The listing builds one solid part. Answer for the finished solid, in the listing's coordinates (mm). Face numbers are marked on the shaded views. A direction names the side the tool comes from. Give positions to 0.01 mm unless a question says otherwise; leave off trailing zeros. Write each loop counter-clockwise with the first axis right and the second up, starting at its lowest first coordinate (ties: lowest second). Pieces come first, ordered by that corner, then holes. Notation, with made-up numbers: (-37.75, 48) -> (-22.75, 48) arc R29 cw to (-22.75, 81) -> close; hole circle Ø2 at (44.5, 2). An arc over 180 degrees is marked (long way). Use CSV: the item, a comma, the result in double quotes. Start each with the question number.
from build123d import *

# Parameters (mm, degrees)
BOSS_EXTRUDE1_DEPTH = 7.5
FILLET1_R           = 5
SKETCH2_W           = 7.7
SKETCH2_H           = 14.7
BOSS_EXTRUDE2_DEPTH = 100
SKETCH3_R           = 2.5
CUT_EXTRUDE1_DEPTH  = 100
SKETCH4_W           = 15
SKETCH4_H           = 60
CUT_EXTRUDE2_DEPTH  = 100
CUT_EXTRUDE3_DEPTH  = 3.75
BOSS_EXTRUDE3_DEPTH = 3.75
SKETCH10_W          = 2.5
SKETCH10_H          = 90
CUT_EXTRUDE4_DEPTH  = 199.475521198


with BuildPart() as part:
    # Sketch1 → Boss-Extrude1 (new, symmetric)
    with BuildSketch(Plane.XY):
        with BuildLine():
            Line((15, 99.936708861), (15, -115.063291139))
            ThreePointArc((15, -115.063291139), (0, -130.063291139), (-15, -115.063291139))
            Line((-15, -115.063291139), (-15, 124.936708861))
            ThreePointArc((-15, 124.936708861), (0, 139.936708861), (15, 124.936708861))
            Line((15, 124.936708861), (25, 124.936708861))
            Line((25, 124.936708861), (25, 99.936708861))
            Line((25, 99.936708861), (15, 99.936708861))
        make_face()
    extrude(amount=BOSS_EXTRUDE1_DEPTH, both=True)

    # Fillet1
    fillet1_edges = [part.edges().sort_by_distance(p)[0] for p in [
        (0, 139.936708861, -7.5),
        (0, -130.063291139, 7.5),
        (15, -7.563291139, 7.5),
        (20, 99.936708861, 7.5),
        (20, 124.936708861, 7.5),
        (0, 139.936708861, 7.5),
        (20, 124.936708861, -7.5),
        (20, 99.936708861, -7.5),
        (15, -7.563291139, -7.5),
        (-15, 4.936708861, 7.5),
        (0, -130.063291139, -7.5),
        (-15, 4.936708861, -7.5),
    ]]
    fillet(fillet1_edges, radius=FILLET1_R)

    # Sketch2 → Boss-Extrude2 (add)
    with BuildSketch(Plane(origin=(25, 0, 0), x_dir=(0, 0, -1), z_dir=(1, 0, 0))):
        with Locations((0, 112.436708861)):
            Rectangle(SKETCH2_W, SKETCH2_H)
    extrude(amount=BOSS_EXTRUDE2_DEPTH)

    # Sketch3 → Cut-Extrude1 (cut)
    with BuildSketch(Plane.XY.offset(3.85)):
        with Locations((35, 112.336708861)):
            Circle(SKETCH3_R)
        with Locations((55, 112.336708861)):
            Circle(SKETCH3_R)
        with Locations((75, 112.336708861)):
            Circle(SKETCH3_R)
        with Locations((95, 112.336708861)):
            Circle(SKETCH3_R)
        with Locations((115, 112.336708861)):
            Circle(SKETCH3_R)
    extrude(amount=-CUT_EXTRUDE1_DEPTH, mode=Mode.SUBTRACT)

    # Sketch4 → Cut-Extrude2 (cut)
    with BuildSketch(Plane.XY.offset(7.5)):
        with Locations((0, -100.063291139)):
            Rectangle(SKETCH4_W, SKETCH4_H)
    extrude(amount=-CUT_EXTRUDE2_DEPTH, mode=Mode.SUBTRACT)

    # Sketch7 → Cut-Extrude3 (cut, symmetric)
    with BuildSketch(Plane(origin=(0, 0, 0), x_dir=(0, 0, -1), z_dir=(1, 0, 0))):
        Polygon((0, 69.936708861), (-7.5, 64.685152324), (-7.5, 74.685152324), (0, 79.936708861), align=None)
        Polygon((0, 49.936708861), (0, 59.936708861), (-7.5, 54.685152324), (-7.5, 44.685152324), align=None)
        Polygon((0, 29.936708861), (0, 39.936708861), (-7.5, 34.685152324), (-7.5, 24.685152324), align=None)
    extrude(amount=CUT_EXTRUDE3_DEPTH, both=True, mode=Mode.SUBTRACT)

    # Sketch8 → Revolve1 (revolve)
    with BuildSketch(Plane.XY):
        with BuildLine():
            Line((-7.5, -113.063291139), (-6, -113.063291139))
            ThreePointArc((-6, -113.063291139), (-6.439339828, -112.002630967), (-7.5, -111.563291139))
            Line((-7.5, -111.563291139), (-7.5, -113.063291139))
        make_face()
        with BuildLine():
            Line((7.5, -113.063291139), (6, -113.063291139))
            ThreePointArc((6, -113.063291139), (6.439339828, -112.002630967), (7.5, -111.563291139))
            Line((7.5, -111.563291139), (7.5, -113.063291139))
        make_face()
    revolve(axis=Axis((-28.138828416, -113.063291139, 0), (1, 0, 0)))

    # Sketch9 → Boss-Extrude3 (add, symmetric)
    with BuildSketch(Plane(origin=(0, 0, 0), x_dir=(0, 0, -1), z_dir=(1, 0, 0))):
        with BuildLine():
            Line((-7.5, 89.436708861), (-7.5, 97.436708861))
            Line((-7.5, 97.436708861), (-14.5, 97.436708861))
            Line((-14.5, 97.436708861), (-14.5, 92.436708861))
            Line((-14.5, 92.436708861), (-10.5, 92.436708861))
            ThreePointArc((-10.5, 92.436708861), (-8.378679656, 91.558029204), (-7.5, 89.436708861))
        make_face()
    extrude(amount=BOSS_EXTRUDE3_DEPTH, both=True)

    # Sketch10 → Cut-Extrude4 (cut, through all)
    with BuildSketch(Plane.ZY.offset(15)):
        with Locations((6.25, -50.063291139)):
            Rectangle(SKETCH10_W, SKETCH10_H)
    extrude(amount=-CUT_EXTRUDE4_DEPTH, mode=Mode.SUBTRACT)


solid = part.part
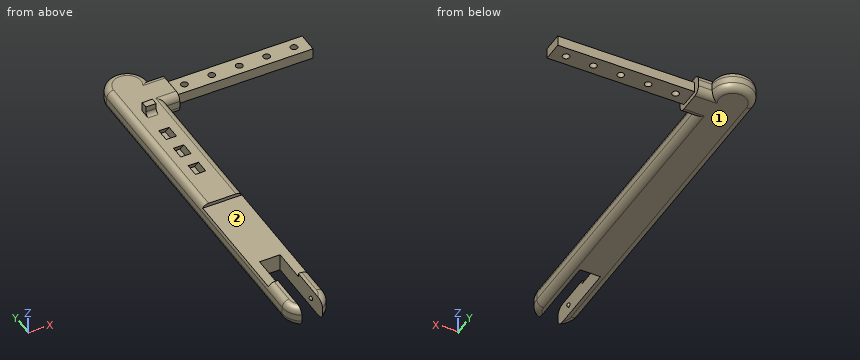
Q1. Straight lines are drawn through the part: L1, parallel to Y at x = 115, z = -2; L2, parallel to X at y = -97.5, z = 2.25; L3, parallel to Z at x = -4, y = -8. For each, find the intervals that lie inside material, in ascending order.
Q2. Section B-B on x = 0 is taken. Give the vertices of the cut face in (y, z), then the cut area to 3 significant figures.
Q3. Section A-A on x = 35 is taken. Give the vertices of the cut face in (y, z).
Q4. Flat-ended cylindrical pins translate along their axes: pin 1 Ø6 at (x, y) = (-1, 35.5) entering from +Z; pin 2 Ø5 at (y, z) = (41, 8) entering from +X; pin 3 Ø5.5 at (y, z) = (92, 12) entering from +X. Find the tip coordinate at first contact, or state that the pin passes through.
Q5. Section C-C on y = 47.5 is taken. Give the vertices of the cut face in (x, z), then the cut area to 3 significant figures.
Q6. For the marked faces 1 and 2, determine the directions among +Z, -Z, +X, -X, +Y, -Y from which every point of the face is accessible in a straight line to the end or side of a thin tool.
Output:
1,L1,"105.09 to 109.84, 114.84 to 119.79"
1,L2,"-15 to -7.5, 7.5 to 15"
1,L3,"-7.5 to 5"
2,outline,"(-70.06, -7.5) -> (134.94, -7.5) arc R5 ccw to (139.94, -2.5) -> (139.94, 2.5) arc R5 ccw to (134.94, 7.5) -> (97.44, 7.5) -> (97.44, 14.5) -> (92.44, 14.5) -> (92.44, 10.5) arc R3 cw to (89.44, 7.5) -> (74.69, 7.5) -> (79.94, 0) -> (69.94, 0) -> (64.69, 7.5) -> (54.69, 7.5) -> (59.94, 0) -> (49.94, 0) -> (44.69, 7.5) -> (34.69, 7.5) -> (39.94, 0) -> (29.94, 0) -> (24.69, 7.5) -> (-5.06, 7.5) -> (-5.06, 5) -> (-70.06, 5) -> close"
2,area,"2,790 mm²"
3,outline,"(105.09, -3.85) -> (109.84, -3.85) -> (109.84, 3.85) -> (105.09, 3.85) -> close; (114.84, -3.85) -> (119.79, -3.85) -> (119.79, 3.85) -> (114.84, 3.85) -> close"
4,pin 1,"z = 7.5"
4,pin 2,"x = 14"
4,pin 3,"x = 3.75"
5,outline,"(-15, -2.5) arc R5 ccw to (-10, -7.5) -> (10, -7.5) arc R5 ccw to (15, -2.5) -> (15, 2.5) arc R5 ccw to (10, 7.5) -> (3.75, 7.5) -> (3.75, 3.48) -> (-3.75, 3.48) -> (-3.75, 7.5) -> (-10, 7.5) arc R5 ccw to (-15, 2.5) -> close"
5,area,"398 mm²"
6,face 1,"-Z, +X, -X, +Y, -Y"
6,face 2,"+Z, +X, -X"
